```python
from build123d import *

# Parameters (mm, degrees)
SKETCH_1_W          = 80
SKETCH_1_H          = 55
EXTRUDE_1_DEPTH     = 1.5
SKETCH_3_R          = 1.6
CUT_EXTRUDE_2_DEPTH = 49.633835958
CUT_EXTRUDE_3_DEPTH = 10


with BuildPart() as part:
    # ｽｹｯﾁ1 → ﾎﾞｽ - 押し出し1 (new, symmetric)
    with BuildSketch(Plane.XY):
        Rectangle(SKETCH_1_W, SKETCH_1_H)
    extrude(amount=EXTRUDE_1_DEPTH, both=True)

    # ｽｹｯﾁ3 → ｶｯﾄ - 押し出し2 (cut, through all)
    with BuildSketch(Plane.XY.offset(1.5)):
        with Locations((-35, 22.5)):
            Circle(SKETCH_3_R)
        with Locations(Location((35, 22.5, 0), (0, 0, 180))):
            Circle(SKETCH_3_R)
        with Locations((35, -22.5)):
            Circle(SKETCH_3_R)
        with Locations(Location((-35, -22.5, 0), (0, 0, 180))):
            Circle(SKETCH_3_R)
    extrude(amount=-CUT_EXTRUDE_2_DEPTH, mode=Mode.SUBTRACT)

    # ｽｹｯﾁ4 → ｶｯﾄ - 押し出し3 (cut)
    with BuildSketch(Plane.XY.offset(1.5)):
        Polygon((30, 27.5), (-30, 27.5), (0, 8.214285714), align=None)
        Polygon((-40, -17.5), (-12.777777778, 0), (-40, 17.5), align=None)
        Polygon((30, -27.5), (0, -8.214285714), (-30, -27.5), align=None)
        Polygon((40, 17.5), (12.777777778, 0), (40, -17.5), align=None)
    extrude(amount=-CUT_EXTRUDE_3_DEPTH, mode=Mode.SUBTRACT)


solid = part.part
```
For this review, take the finished solid that the model builds, in its own axes (mm). A direction names the side the tool comes from. Give positions to 0.01 mm unless a question says otherwise; leave off trailing zeros. Order: outer loops, then holes, each group sorted by start corner. A loop starts at its lowest first (then second) coordinate and runs counter-clockwise, first axis right, second up.
1) Insertion check: pin 1 (4 mm diameter, centred on x = -35, y = 22.5, fed in from -Z); pin 2 (1.9 mm diameter, centred on x = -35, y = -22.5, fed in from +Z). Each pin has a flat end and moves straight along its axis. Give the tip position at first contact, or say it passes through.
2) Take a section at B-B (y = -19). Give the boundary of the cut face in (x, z), then the cut area to 3 significant figures.
3) For faces 1 (the face through (14.79, 17.72, 0.02)), 2 (the face through (15.21, -17.99, 0.02)), 3 (the face through (-26.579, -8.872, 0.021)), 4 (the face through (35, -27.5, 0)), list the 3-axis set-ups (+Z, -Z, +X, -X, +Y, -Y) from which the entire face can be reached by the end or side of a thin tool; tool diameter is ignored.
4) Take a section at D-D (x = -32). Give the boundary of the cut face in (y, z).
5) Wall thickness on line 1 (Y direction, x = 34, z = -0.3); line 2 (Y direction, x = -35, z = 0.75); line 3 (X direction, y = 15, z = 0.45): over which ranges is each line inside the solid? List them lowest first.
6) Take a section at A-A (x = 35). Give the boundary of the cut face in (y, z).
7) Take a section at C-C (z = -0.55). Give the boundary of the cut face in (x, y), then the cut area to 3 significant figures.
8) The part is to be moulded in two halves that separate along X. For faces 5 (the face through (-26.2, 8.63, 0.02)), 6 (the face through (26.579, 8.872, 0.021)), 7 (the face through (-15.21, 17.99, 0.02)), say which applies: released by +X, released by -X, zero draft, split by the parting line, or undercut.
Derived:
1. pin 1: stops at z = -1.5
1. pin 2: passes through
2. outline: (-40, -1.5) - (-16.78, -1.5) - (-16.78, 1.5) - (-40, 1.5) - close; (16.78, -1.5) - (40, -1.5) - (40, 1.5) - (16.78, 1.5) - close
2. area: 139 mm2
3. face 1: +Z, -Z, +Y
3. face 2: +Z, -Z, -Y
3. face 3: +Z, -Z, -X
3. face 4: +Z, -Z, +X, -X, -Y
4. outline: (-27.5, -1.5) - (-12.36, -1.5) - (-12.36, 1.5) - (-27.5, 1.5) - close; (12.36, -1.5) - (27.5, -1.5) - (27.5, 1.5) - (12.36, 1.5) - close
5. line 1: y = -27.5 to -23.75, -21.25 to -13.64, 13.64 to 21.25, 23.75 to 27.5
5. line 2: y = -27.5 to -24.1, -20.9 to -14.29, 14.29 to 20.9, 24.1 to 27.5
5. line 3: x = -36.11 to -10.56, 10.56 to 36.11
6. outline: (-27.5, -1.5) - (-24.1, -1.5) - (-24.1, 1.5) - (-27.5, 1.5) - close; (-20.9, -1.5) - (-14.29, -1.5) - (-14.29, 1.5) - (-20.9, 1.5) - close; (14.29, -1.5) - (20.9, -1.5) - (20.9, 1.5) - (14.29, 1.5) - close; (24.1, -1.5) - (27.5, -1.5) - (27.5, 1.5) - (24.1, 1.5) - close
7. outline: (-40, -27.5) - (-30, -27.5) - (0, -8.21) - (30, -27.5) - (40, -27.5) - (40, -17.5) - (12.78, 0) - (40, 17.5) - (40, 27.5) - (30, 27.5) - (0, 8.21) - (-30, 27.5) - (-40, 27.5) - (-40, 17.5) - (-12.78, 0) - (-40, -17.5) - close; hole circle Ø3.2 at (-35, -22.5); hole circle Ø3.2 at (-35, 22.5); hole circle Ø3.2 at (35, -22.5); hole circle Ø3.2 at (35, 22.5)
7. area: 2,260 mm2
8. face 5: released by -X
8. face 6: released by +X
8. face 7: undercut
